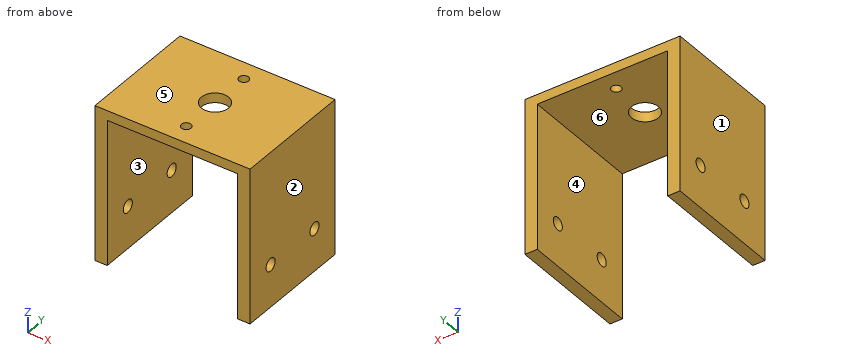
from build123d import *

# Parameters (mm, degrees)
SKETCH3_W           = 33.65
SKETCH3_H           = 31
SKETCH3_R           = 1.25
SKETCH3_R_2         = 3.5
BOSS_EXTRUDE3_DEPTH = 2.5
SKETCH3_3_W         = 3.175
SKETCH3_3_H         = 31
BOSS_EXTRUDE4_DEPTH = 40
SKETCH4_R           = 1.65
CUT_EXTRUDE1_DEPTH  = 40


with BuildPart() as part:
    # Sketch3 → Boss-Extrude3 (new body)
    with BuildSketch(Plane.XY):
        with Locations((0, 15.5)):
            Rectangle(SKETCH3_W, SKETCH3_H)
        with Locations((0, 5)):
            Circle(SKETCH3_R, mode=Mode.SUBTRACT)
        with Locations((0, 15.5)):
            Circle(SKETCH3_R_2, mode=Mode.SUBTRACT)
        with Locations((0, 26)):
            Circle(SKETCH3_R, mode=Mode.SUBTRACT)
    extrude(amount=-BOSS_EXTRUDE3_DEPTH)

    # Sketch3<3> → Boss-Extrude4 (add)
    with BuildSketch(Plane.XY):
        with Locations((-18.4125, 15.5)):
            Rectangle(SKETCH3_3_W, SKETCH3_3_H)
        with Locations((18.4125, 15.5)):
            Rectangle(SKETCH3_3_W, SKETCH3_3_H)
    extrude(amount=-BOSS_EXTRUDE4_DEPTH)

    # Sketch4 → Cut-Extrude1 (cut)
    with BuildSketch(Plane.ZY.offset(20)):
        with Locations((-29.03, 23.5)):
            Circle(SKETCH4_R)
        with Locations((-29.03, 7.5)):
            Circle(SKETCH4_R)
    extrude(amount=-CUT_EXTRUDE1_DEPTH, mode=Mode.SUBTRACT)


solid = part.part
Input: part model. Units: mm. Frame: model coordinates. Face numbers are marked on the shaded views. A direction names the side the tool comes from. Coordinates: 2 decimals unless noted, no trailing zeros. Write each loop counter-clockwise with the first axis right and the second up, starting at its lowest first coordinate (ties: lowest second). Pieces come first, ordered by that corner, then holes. Notation, with made-up numbers: M 8,-10 L 53,-10 A14 cw 53,8 Z; hole C 27,50.25 d4. An arc over 180 degrees is marked long. Answer as a JSON object with one key per item and string values. Group by question number.
(1) Mould query, pull axis X, two halves, no side actions, for the marked faces 1, 2, 3 and 4. Classes: pulls with the +X half, pulls with the -X half, needs draft (parallel to the pull), parting line crosses it, or undercut.
(2) Set-up query: the marked faces 5 and 6. Return all of +Z, -Z, +X, -X, +Y, -Y with unobstructed straight access to the full face (end or side cutting, diameter ignored); none if empty.
(3) Section C-C on y = 15.5. Output: boundary loops of the cut face in (x, z) (3 decimals), plus the area to 3 significant figures.
(4) Ray query, line 1 along Y through (x, z) = (18.45, -29.03); line 2 along X through (y, z) = (14.5, -11) (3 decimals); line 3 along Z through (x, y) = (-12.5, 23). Return the intervals inside material, ascending. Write a range as [from, to].
(5) Contact query for a flat-ended pin moving along its axis: P1, Ø1, axis at x = 9.5, y = 6.5, coming from the -Z side. Output: stop coordinate, or through.
(6) Section A-A on z = -15. Output: boundary loops of the cut face in (x, y) (3 decimals), plus the area to 3 significant figures.
(7) Section B-B on x = 0. Output: boundary loops of the cut face in (y, z), plus the area to 3 significant figures.
(8) Section D-D on z = -29.03. Output: boundary loops of the cut face in (x, y) (3 decimals).
Result set:
{
 "1": {"face 1": "pulls with the -X half", "face 2": "pulls with the +X half", "face 3": "undercut", "face 4": "undercut"},
 "2": {"face 5": "+Z, +X, -X, +Y, -Y", "face 6": "-Z, +Y, -Y"},
 "3": {"outline": "M -20,-40 L -16.825,-40 L -16.825,-2.5 L -3.5,-2.5 L -3.5,0 L -20,0 Z; M 3.5,-2.5 L 16.825,-2.5 L 16.825,-40 L 20,-40 L 20,0 L 3.5,0 Z", "area": "321 mm2"},
 "4": {"line 1": "y = [0, 5.85], [9.15, 21.85], [25.15, 31]", "line 2": "x = [-20, -16.825], [16.825, 20]", "line 3": "z = [-2.5, 0]"},
 "5": {"P1": "stops at z = -2.5"},
 "6": {"outline": "M -20,0 L -16.825,0 L -16.825,31 L -20,31 Z; M 16.825,0 L 20,0 L 20,31 L 16.825,31 Z", "area": "197 mm2"},
 "7": {"outline": "M 0,-2.5 L 3.75,-2.5 L 3.75,0 L 0,0 Z; M 6.25,-2.5 L 12,-2.5 L 12,0 L 6.25,0 Z; M 19,-2.5 L 24.75,-2.5 L 24.75,0 L 19,0 Z; M 27.25,-2.5 L 31,-2.5 L 31,0 L 27.25,0 Z", "area": "47.5 mm2"},
 "8": {"outline": "M -20,0 L -16.825,0 L -16.825,5.85 L -20,5.85 Z; M -20,9.15 L -16.825,9.15 L -16.825,21.85 L -20,21.85 Z; M -20,25.15 L -16.825,25.15 L -16.825,31 L -20,31 Z; M 16.825,0 L 20,0 L 20,5.85 L 16.825,5.85 Z; M 16.825,9.15 L 20,9.15 L 20,21.85 L 16.825,21.85 Z; M 16.825,25.15 L 20,25.15 L 20,31 L 16.825,31 Z"}
}
